Source: three-view drawing plus pictorial views. Frame: mm from the lowest corner of the part. A direction names the side the tool comes from. Round coordinates to 2 decimals unless told otherwise and drop trailing zeros. Write each loop counter-clockwise with the first axis right and the second up, starting at its lowest first coordinate (ties: lowest second). Pieces come first, ordered by that corner, then holes. Notation, with made-up numbers: (25, 12.25) -> (56, 12.25) arc R22 cw to (56, 21.25) -> close; hole circle Ø5 at (46.5, 81). An arc over 180 degrees is marked (long way). Put each result on its own line as item: value.
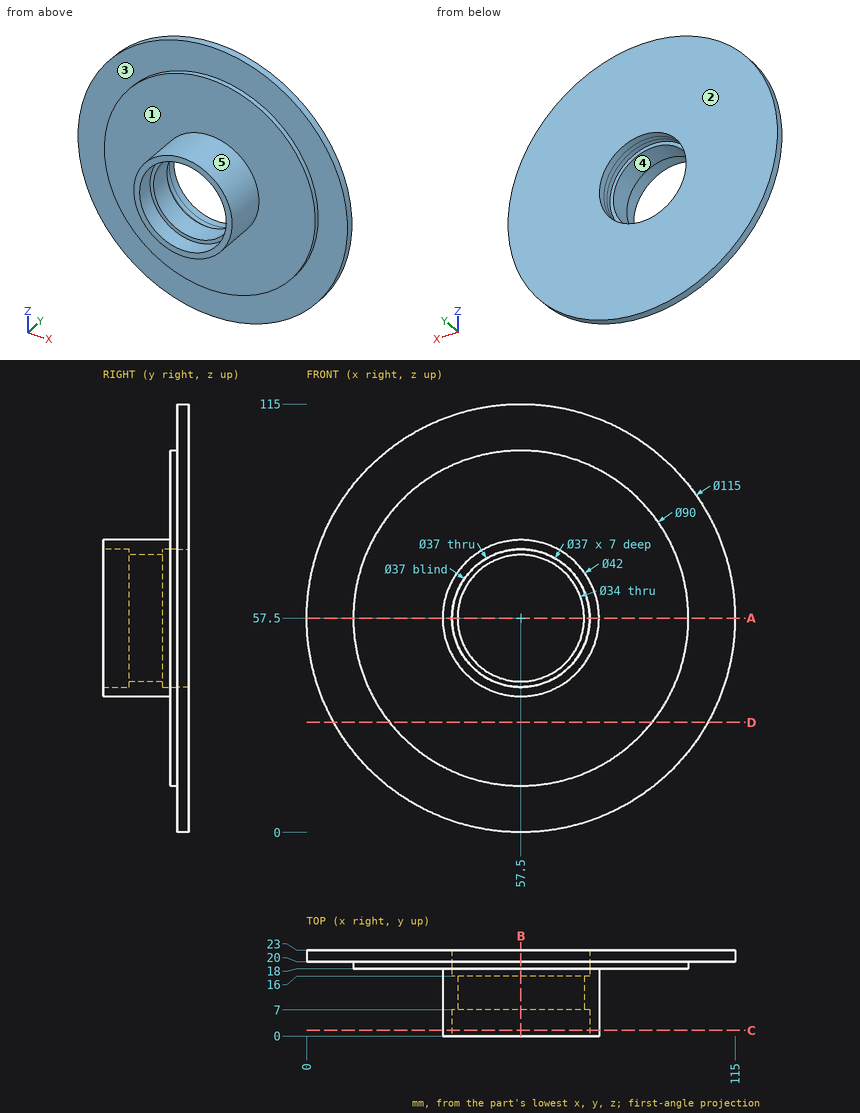
Q1. Pin query (flat end, axial travel): pin 1 (1.5 mm diameter, centred on y = 20.5, z = 36, fed in from -X); pin 2 (1 mm diameter, centred on x = 16.5, z = 83.5, fed in from -Y); pin 3 (20.5 mm diameter, centred on x = 57.5, z = 57.5, fed in from +Y); pin 4 (3 mm diameter, centred on x = 71, y = 2.5, fed in from +Z). Return the tip coordinate at first contact, or that it passes through.
Ans:
pin 1: stops at x = 3.87
pin 2: stops at y = 20
pin 3: passes through
pin 4: stops at z = 74.73
Q2. Cut plane D-D on z = 29.5. Output: boundary loops of the cut face in (x, y), and give its area (3 significant figures).
Ans:
outline: (7.28, 20) -> (22.27, 20) -> (22.27, 18) -> (92.73, 18) -> (92.73, 20) -> (107.72, 20) -> (107.72, 23) -> (7.28, 23) -> close
area: 442 mm^2
Q3. Draft query along Z for the marked faces 3, 4 and 5. Return one class per face: +Z half, -Z half, draft (parallel to the pull), parting line (faces both ways), or undercut.
Ans:
face 3: draft
face 4: undercut
face 5: parting line
Q4. Reachability of the marked faces 1 and 2 from +Z, -Z, +X, -X, +Y, -Y: full face, straight path, thin tool, end or side. Return the list, or none.
Ans:
face 1: -Y
face 2: +Z, -Z, +X, -X, +Y
Q5. Cut plane C-C on y = 1.5. Output: boundary loops of the cut face in (x, z).
Ans:
outline: circle Ø42 at (57.5, 57.5); hole circle Ø37 at (57.5, 57.5)
Q6. Cut plane B-B on x = 57.5. Output: boundary loops of the cut face in (y, z).
Ans:
outline: (0, 36.5) -> (18, 36.5) -> (18, 12.5) -> (20, 12.5) -> (20, 0) -> (23, 0) -> (23, 39) -> (16, 39) -> (16, 40.5) -> (7, 40.5) -> (7, 39) -> (0, 39) -> close; (0, 76) -> (7, 76) -> (7, 74.5) -> (16, 74.5) -> (16, 76) -> (23, 76) -> (23, 115) -> (20, 115) -> (20, 102.5) -> (18, 102.5) -> (18, 78.5) -> (0, 78.5) -> close
Q7. Material intervals for line 1 (X direction, y = 18.8, z = 57.5); line 2 (X direction, y = 13.5, z = 57.5); line 3 (Y direction, x = 18.5, z = 65.5), sorted ascending. Write a range as [from, to].
Ans:
line 1: x = [12.5, 39], [76, 102.5]
line 2: x = [36.5, 40.5], [74.5, 78.5]
line 3: y = [18, 23]
Q8. Cut plane A-A on z = 57.5. Output: boundary loops of the cut face in (x, y), and give its area (3 significant figures).
Ans:
outline: (0, 20) -> (12.5, 20) -> (12.5, 18) -> (36.5, 18) -> (36.5, 0) -> (39, 0) -> (39, 7) -> (40.5, 7) -> (40.5, 16) -> (39, 16) -> (39, 23) -> (0, 23) -> close; (74.5, 7) -> (76, 7) -> (76, 0) -> (78.5, 0) -> (78.5, 18) -> (102.5, 18) -> (102.5, 20) -> (115, 20) -> (115, 23) -> (76, 23) -> (76, 16) -> (74.5, 16) -> close
area: 457 mm^2
